Design review of the part built by this model. Coordinates are the model's own, in mm. Face numbers are marked on the shaded views. A direction names the side the tool comes from. Give positions to 0.01 mm unless a question says otherwise; leave off trailing zeros. Write each loop counter-clockwise with the first axis right and the second up, starting at its lowest first coordinate (ties: lowest second). Pieces come first, ordered by that corner, then holes. Notation, with made-up numbers: (85, 35.5) -> (109, 35.5) arc R24 cw to (109, 53.5) -> close; hole circle Ø10 at (38, -2.5). An arc over 180 degrees is marked (long way). Return JSON: item names as keys, results as strings. Group by question number.
Autodesk Inventor part; units mm, degrees
ref_plane "YZ Plane" through (0, 0, 0) normal (1, 0, 0) x (0, 1, 0)
ref_plane "XZ Plane" through (0, 0, 0) normal (0, 1, 0) x (-1, 0, 0)
ref_plane "XY Plane" through (0, 0, 0) normal (0, 0, 1) x (1, 0, 0)
sketch "Sketch1" plane through (0, 0, 0) normal (1, 0, 0) x (0, 1, 0)
  line L0 (-1.8333, 27.5) -> (1.8333, 27.5)
  line L1 (1.8333, -27.5) -> (-1.8333, -27.5)
  line L2 (-1.8333, -27.5) -> (-1.8333, 27.5)
  line L3 (-1.8333, 27.5) -> (1.8333, -27.5) construction
  line L4 (1.8333, 27.5) -> (-1.8333, -27.5) construction
  arc A0 (12.6667, -14.5) -> (12.6667, 14.5) centre (12.6667, 0) ccw
  line L5 (12.6667, 14.5) -> (1.8333, 14.5)
  line L6 (12.6667, -14.5) -> (1.8333, -14.5)
  circle A1 centre (12.6667, 0) radius 4
  line L7 (1.8333, 27.5) -> (1.8333, 14.5)
  line L8 (1.8333, -14.5) -> (1.8333, -27.5)
  point P0 (0, 0)
  dimension "d0" = 55
  dimension "d2" = 8
extrude "Extrusion1" add sketch "Sketch1" along normal blind 13
sketch "Sketch2" plane through (0, 1.8333, 27.5) normal (0, 1, 0) x (1, 0, 0)
  line L0 (13, 13) -> (13, 42)
  line L1 (0, 0) -> (13, 13) construction
  line L2 (0, 55) -> (0, 0)
  line L3 (0, 42) -> (13, 42)
  line L4 (0, 55) -> (13, 42) construction
  circle A0 centre (6.5, 6.5) radius 2.5
  circle A1 centre (6.5, 48.5) radius 2.5
  point P0 (0, 27.5)
  dimension "d5" = 5
  dimension "d6" = 5
extrude "Extrusion2" cut sketch "Sketch2" against normal blind 13
properties part number "bearingStandin" material "Gold"
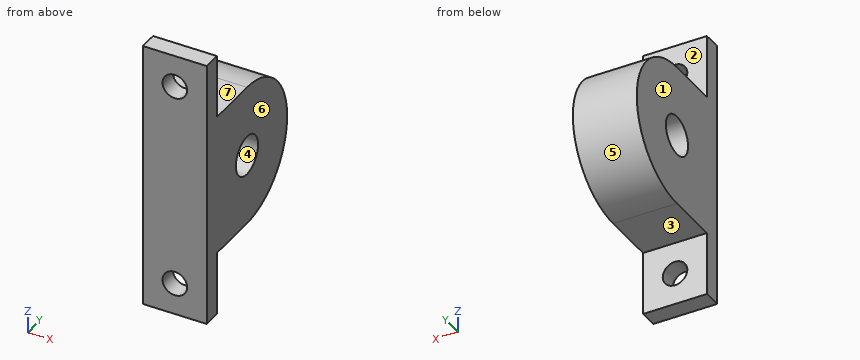
Q1. Tool access review of the marked faces 1, 2 and 3: name each direction out of +Z, -Z, +X, -X, +Y, -Y from which nothing blocks a thin tool from reaching the whole face with its end or side.
Q2. Insertion check: pin 1 (6 mm diameter, centred on x = 10.5, z = 8, fed in from +Y); pin 2 (5.5 mm diameter, centred on x = 7.5, y = 5.5, fed in from +Z); pin 3 (5 mm diameter, centred on x = 7, z = -12, fed in from +Y). Each pin has a flat end and moves straight along its axis. Give the tip position at first contact, or say it passes through.
Q3. Take a section at C-C, the plane y = 0.25. Give the boundary of the cut face in (x, z), plus the area to 3 significant figures.
Q4. Take a section at A-A, the plane x = 5. Give the boundary of the cut face in (y, z), plus the area to 3 significant figures.
Q5. Mouldability with a two-part tool opening along Z and no side actions: class the marked faces 4, 5, 6 and 7 as +Z half, -Z half, draft (parallel to the pull), parting line (faces both ways), or undercut.
Q6. For L1, parallel to Z at x = 6.5, y = 0.85; L2, parallel to Z at x = 11.25, y = 12.5; L3, parallel to X at y = -1, z = 21, list the stretches that pass through material, from the lowest coordinate up. Write a range as from..to.
Q7. Take a section at B-B, the plane z = 0. Give the boundary of the cut face in (x, y), plus the area to 3 significant figures.
Q8. Take a section at D-D, the plane x = 1. Give the boundary of the cut face in (y, z), plus the area to 3 significant figures.
Final values:
{
 "1": {"face 1": "+Z, -Z, -X, +Y, -Y", "face 2": "+Z, +X, -X, +Y", "face 3": "-Z, +X, -X, +Y"},
 "2": {"pin 1": "stops at y = 26.28", "pin 2": "stops at z = 14.5", "pin 3": "stops at y = 23.62"},
 "3": {"outline": "(0, -27.5) -> (13, -27.5) -> (13, 27.5) -> (0, 27.5) -> close; hole circle Ø5 at (6.5, -21); hole circle Ø5 at (6.5, 21)", "area": "676 mm²"},
 "4": {"outline": "(-1.83, -27.5) -> (1.83, -27.5) -> (1.83, -23) -> (-1.83, -23) -> close; (-1.83, -19) -> (1.83, -19) -> (1.83, -14.5) -> (12.67, -14.5) arc R14.5 ccw to (12.67, 14.5) -> (1.83, 14.5) -> (1.83, 19) -> (-1.83, 19) -> close; (-1.83, 23) -> (1.83, 23) -> (1.83, 27.5) -> (-1.83, 27.5) -> close; hole circle Ø8 at (12.67, 0)", "area": "766 mm²"},
 "5": {"face 4": "undercut", "face 5": "parting line", "face 6": "draft", "face 7": "+Z half"},
 "6": {"L1": "z = -27.5..-23.5, -18.5..18.5, 23.5..27.5", "L2": "z = -14.5..-4, 4..14.5", "L3": "x = 0..4, 9..13"},
 "7": {"outline": "(0, -1.83) -> (13, -1.83) -> (13, 8.67) -> (0, 8.67) -> close; (0, 16.67) -> (13, 16.67) -> (13, 27.17) -> (0, 27.17) -> close", "area": "273 mm²"},
 "8": {"outline": "(-1.83, -27.5) -> (1.83, -27.5) -> (1.83, -14.5) -> (12.67, -14.5) arc R14.5 ccw to (12.67, 14.5) -> (1.83, 14.5) -> (1.83, 27.5) -> (-1.83, 27.5) -> close; hole circle Ø8 at (12.67, 0)", "area": "796 mm²"}
}
